The listing builds one solid part. Answer for the finished solid, in the listing's coordinates (mm). Round coordinates to 2 decimals unless told otherwise and drop trailing zeros. Write each loop counter-clockwise with the first axis right and the second up, starting at its lowest first coordinate (ties: lowest second). Pieces come first, ordered by that corner, then holes. Notation, with made-up numbers: (-22, 66.25) - (4, 66.25) arc R12 ccw to (4, 83.25) - close; hole circle Ø4 at (61, -9). An arc over 180 degrees is marked (long way). Return JSON: item names as keys, results as strings. Group by question number.
(1) Section C-C, the plane x = 4.4 is taken. Write down the section's boundary in (y, z).
(2) Each of these flat-tipped pins is pushed along its axis until it touches: pin 1 (2 mm diameter, centred on x = 4, z = 53, fed in from +Y); pin 2 (18 mm diameter, centred on y = 92, z = 27.5, fed in from +X); pin 3 (1.8 mm diameter, centred on x = 1.5, y = 138, fed in from +Z); pin 4 (3 mm diameter, centred on x = 2.5, z = 53.5, fed in from -Y). Where does it stop, or does it pass through?
(3) Find the intervals of material crossed by line 1 along Z through (x, y) = (1.6, 40); line 2 along Y through (x, z) = (4.15, 35); line 3 along Y through (x, z) = (4.25, 38), in increasing order. Write a range as [from, to].
(4) Section D-D, the plane y = 135.5 is taken. Write down the section's boundary in (x, z), then the cut area to 3 significant figures.
(5) Section A-A, the plane z = 27.5 is taken. Write down the section's boundary in (x, y), then the cut area to 3 significant figures.
(6) Section B-B, the plane y = 40 is taken. Write down the section's boundary in (x, z), then the cut area to 3 significant figures.
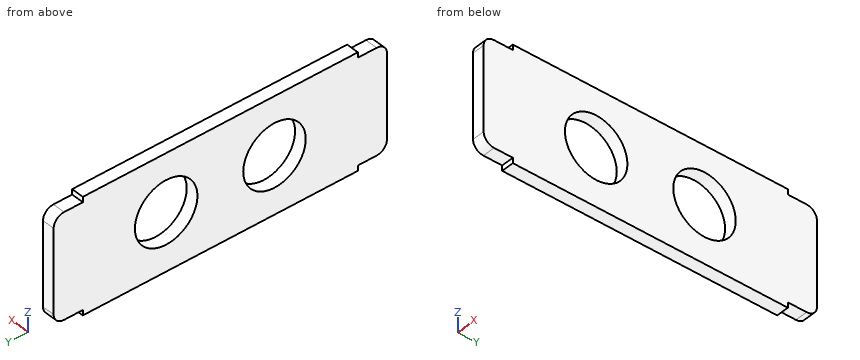
```python
from build123d import *

# Parameters (mm, degrees)
F0_R     = 15
F0_W     = 14
F0_H     = 50
F1_DEPTH = 6
F2_R     = 5


with BuildPart() as f1:
    # F0 (on Right) → F1 (new body)
    with BuildSketch(Plane.YZ):
        Polygon((132, 55), (0, 55), (0, 52.5), (0, 2.5), (0, 0), (132, 0), (132, 2.5), (132, 52.5), align=None)
        with Locations((40, 27.5)):
            Circle(F0_R, mode=Mode.SUBTRACT)
        with Locations((92, 27.5)):
            Circle(F0_R, mode=Mode.SUBTRACT)
        with Locations((-7, 27.5)):
            Rectangle(F0_W, F0_H)
        with Locations((139, 27.5)):
            Rectangle(F0_W, F0_H)
    extrude(amount=F1_DEPTH)

    # F2
    f2_edges = [f1.edges().sort_by_distance(p)[0] for p in [
        (3, -14, 2.5),
        (3, -14, 52.5),
        (3, 146, 52.5),
        (3, 146, 2.5),
    ]]
    fillet(f2_edges, radius=F2_R)


solid = f1.part
```
Working result:
{
 "1": {"outline": "(-14, 7.5) arc R5 ccw to (-9, 2.5) - (0, 2.5) - (0, 0) - (132, 0) - (132, 2.5) - (141, 2.5) arc R5 ccw to (146, 7.5) - (146, 47.5) arc R5 ccw to (141, 52.5) - (132, 52.5) - (132, 55) - (0, 55) - (0, 52.5) - (-9, 52.5) arc R5 ccw to (-14, 47.5) - close; hole circle Ø30 at (40, 27.5); hole circle Ø30 at (92, 27.5)"},
 "2": {"pin 1": "stops at y = 143.18", "pin 2": "passes through", "pin 3": "stops at z = 52.5", "pin 4": "stops at y = -11.18"},
 "3": {"line 1": "z = [0, 12.5], [42.5, 55]", "line 2": "y = [-14, 27.01], [52.99, 79.01], [104.99, 146]", "line 3": "y = [-14, 29.29], [50.71, 81.29], [102.71, 146]"},
 "4": {"outline": "(0, 2.5) - (6, 2.5) - (6, 52.5) - (0, 52.5) - close", "area": "300 mm^2"},
 "5": {"outline": "(0, -14) - (6, -14) - (6, 25) - (0, 25) - close; (0, 55) - (6, 55) - (6, 77) - (0, 77) - close; (0, 107) - (6, 107) - (6, 146) - (0, 146) - close", "area": "600 mm^2"},
 "6": {"outline": "(0, 0) - (6, 0) - (6, 12.5) - (0, 12.5) - close; (0, 42.5) - (6, 42.5) - (6, 55) - (0, 55) - close", "area": "150 mm^2"}
}
